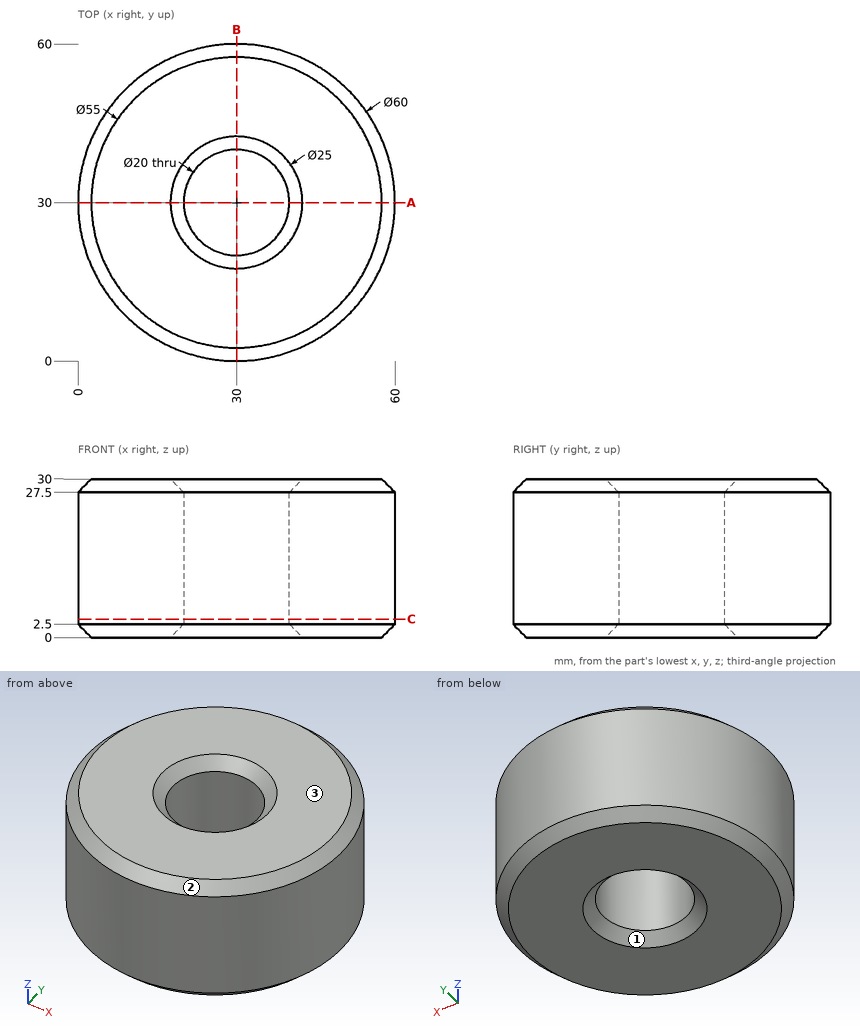
The drawing under review shows one solid part. Ordinate dimensions are in mm from its lowest x, y, z. Round coordinates to 2 decimals unless told otherwise and drop trailing zeros. Loops run counter-clockwise (first coordinate to the right, second up) from the corner with the lowest first, then second, coordinate; pieces in that order, holes last. Notation, with made-up numbers: M 41,5.5 L 46,5.5 A23 cw 46,35.5 Z; hole C -2.5,9.25 d11. An arc over 180 degrees is marked long. Answer as CSV lines item,"result". Start each with the question number.
Item 1: Wall thickness on line 1 (Y direction, x = 30, z = 8); line 2 (X direction, y = 42, z = 23.25): over which ranges is each line inside the solid? List them lowest first. Write a range as [from, to].
Item 2: Mouldability with a two-part tool opening along X and no side actions: class the marked faces 1, 2 and 3 as released by +X, released by -X, zero draft, split by the parting line, or undercut.
Item 3: Consider section A-A (y = 30). Write out the cut boundary in (x, z), then the cut area to 4 significant figures.
Item 4: Consider section C-C (z = 3.5). Write out the cut boundary in (x, y).
Item 5: Insertion check: P1, Ø10, axis at y = 35.5, z = 10.5, coming from the -X side; P2, Ø3, axis at x = 38, z = 11, coming from the +Y side; P3, Ø18, axis at x = 30, y = 30, coming from the -Z side; P4, Ø8, axis at x = 11, z = 17.5, coming from the +Y side. Each pin has a flat end and moves straight along its axis. Give the tip position at first contact, or say it passes through.
Answer:
1,line 1,"y = [0, 20], [40, 60]"
1,line 2,"x = [2.5, 57.5]"
2,face 1,"undercut"
2,face 2,"split by the parting line"
2,face 3,"zero draft"
3,outline,"M 0,2.5 L 2.5,0 L 17.5,0 L 20,2.5 L 20,27.5 L 17.5,30 L 2.5,30 L 0,27.5 Z; M 40,2.5 L 42.5,0 L 57.5,0 L 60,2.5 L 60,27.5 L 57.5,30 L 42.5,30 L 40,27.5 Z"
3,area,"1,175 mm^2"
4,outline,"C 30,30 d60; hole C 30,30 d20"
5,P1,"stops at x = 0"
5,P2,"stops at y = 59.29"
5,P3,"passes through"
5,P4,"stops at y = 55.98"
